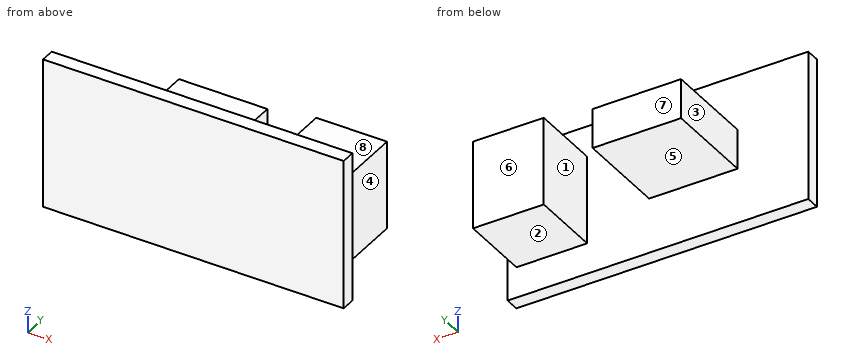
```python
from build123d import *

# Parameters (mm, degrees)
SKETCH1_W            = 34
SKETCH1_H            = 17
BOARD_DEPTH          = 1.6
TO220_START          = 1.6
SKETCH2_W            = 10
SKETCH2_H            = 4.5
TO220_DEPTH          = 10.4
TERMINAL_BLOCK_START = 1.6
SKETCH3_W            = 8
SKETCH3_H            = 10
TERMINAL_BLOCK_DEPTH = 8


with BuildPart() as part:
    # Sketch1 → Board (new body)
    with BuildSketch(Plane(origin=(0, 0, 0), x_dir=(1, 0, 0), z_dir=(0, 1, 0))):
        Rectangle(SKETCH1_W, SKETCH1_H)
    extrude(amount=BOARD_DEPTH)

    # Sketch2 → TO220 (add)
    with BuildSketch(Plane(origin=(0, 0, 0), x_dir=(1, 0, 0), z_dir=(0, 1, 0)).offset(TO220_START)):
        with Locations((-4, 0)):
            Rectangle(SKETCH2_W, SKETCH2_H)
    extrude(amount=TO220_DEPTH)

    # Sketch3 → Terminal_Block (add)
    with BuildSketch(Plane(origin=(0, 0, 0), x_dir=(1, 0, 0), z_dir=(0, 1, 0)).offset(TERMINAL_BLOCK_START)):
        with Locations((12, 0)):
            Rectangle(SKETCH3_W, SKETCH3_H)
    extrude(amount=TERMINAL_BLOCK_DEPTH)


solid = part.part
```
Model file for the job. Use its own axes, mm. Face numbers are marked on the shaded views. A direction names the side the tool comes from. Round coordinates to 2 decimals unless told otherwise and drop trailing zeros. Write each loop counter-clockwise with the first axis right and the second up, starting at its lowest first coordinate (ties: lowest second). Pieces come first, ordered by that corner, then holes. Notation, with made-up numbers: (65, 73) - (78, 73) arc R25 cw to (78, 107) - close; hole circle Ø11 at (8.5, 58). An arc over 180 degrees is marked (long way). One line per item, written item: value.
(1) Drop flat-ended pins along their axis: P1, Ø3, axis at x = -2.5, y = 4.5, coming from the +Z side; P2, Ø2, axis at y = 5, z = 0, coming from the +X side; P3, Ø9, axis at x = 11.5, z = -1.5, coming from the +Y side. Give the stop position or say it passes through.
Values follow:
P1: stops at z = 2.25
P2: stops at x = 16
P3: stops at y = 9.6
(2) 3-axis set-ups, long thin cutter, end or side, ignore diameter. For the marked faces 5, 6, 7 and 8: which of +Z, -Z, +X, -X, +Y, -Y reach the whole face in a straight line?
Values follow:
face 5: -Z, -X, +Y
face 6: +Z, -Z, +X, +Y
face 7: +Z, -Z, +X, -X, +Y
face 8: +Z, +X, -X, +Y
(3) Cut at D-D, the plane x = 10. Give the cut face in (y, z).
Values follow:
outline: (0, -8.5) - (1.6, -8.5) - (1.6, -5) - (9.6, -5) - (9.6, 5) - (1.6, 5) - (1.6, 8.5) - (0, 8.5) - close
(4) Cut at C-C, the plane z = -0.25. Give the cut face in (x, y), plus the area to 3 significant figures.
Values follow:
outline: (-17, 0) - (17, 0) - (17, 1.6) - (16, 1.6) - (16, 9.6) - (8, 9.6) - (8, 1.6) - (1, 1.6) - (1, 12) - (-9, 12) - (-9, 1.6) - (-17, 1.6) - close
area: 222 mm²
(5) Cut at B-B, the plane x = -1. Give the cut face in (y, z), plus the area to 3 significant figures.
Values follow:
outline: (0, -8.5) - (1.6, -8.5) - (1.6, -2.25) - (12, -2.25) - (12, 2.25) - (1.6, 2.25) - (1.6, 8.5) - (0, 8.5) - close
area: 74.0 mm²
(6) Two-plate mould, pull along X, no slides. Class the marked faces 1, 2, 3 and 4: pulls with the +X half, pulls with the -X half, needs draft (parallel to the pull), parting line crosses it, or undercut.
Values follow:
face 1: undercut
face 2: needs draft
face 3: pulls with the -X half
face 4: pulls with the +X half
(7) Wall check: probe 1 along X at (y, z) = (8.25, 1.5); probe 2 along Z at (x, y) = (13.5, 6.5); probe 3 along Z at (x, y) = (-1, 1.75). Give the ranges that are in metal, low to high.
Values follow:
probe 1: x = -9 to 1, 8 to 16
probe 2: z = -5 to 5
probe 3: z = -2.25 to 2.25
(8) Cut at A-A, the plane y = 3. Give the cut face in (x, z).
Values follow:
outline: (-9, -2.25) - (1, -2.25) - (1, 2.25) - (-9, 2.25) - close; (8, -5) - (16, -5) - (16, 5) - (8, 5) - close
